Model file for the job. Use its own axes, mm. A direction names the side the tool comes from. Round coordinates to 2 decimals unless told otherwise and drop trailing zeros. Loops run counter-clockwise (first coordinate to the right, second up) from the corner with the lowest first, then second, coordinate; pieces in that order, holes last. Notation, with made-up numbers: M 61,-32.5 L 112,-32.5 A18 cw 112,-23.5 Z; hole C -19.5,52 d9. An arc over 180 degrees is marked long. Use a Markdown table: item, result. Add a question column.
Q1. Tool access for faces 1 (the face through (-1, 9, 75)), 2 (the face through (-1, 8, 77)): list every direction of +Z, -Z, +X, -X, +Y, -Y with a clear straight run to the whole face (end or side of a thin tool).
Q2. Cut at C-C (y = 5.5). Give the cut face in (x, z).
Q3. Cut at B-B (x = 31). Give the cut face in (y, z).
Q4. Probe line 1 (X direction, y = 15.5, z = 20.5); line 2 (Y direction, x = 62.5, z = 6). List the from-to ranges inside material, lowest first. Write a range as from..to.
Q5. Cut at A-A (z = -65.5). Give the cut face in (x, y), plus the area to 3 significant figures.
Q6. Mould opens along Z. For faces 3 (the face through (-1, 0, -1)), 4 (the face through (-1, 9, -75)), 5 (the face through (-1, 2, -1)), 6 (the face through (-1, 8, -77)) say: +Z half, -Z half, draft (parallel to the pull), parting line (faces both ways), or undercut.
from build123d import *

# Parameters (mm, degrees)
SKETCH1_W           = 150
SKETCH1_H           = 150
BOSS_EXTRUDE1_DEPTH = 2
SKETCH2_W           = 154
SKETCH2_H           = 154
BOSS_EXTRUDE2_DEPTH = 2
SKETCH3_W           = 154
SKETCH3_H           = 154
SKETCH3_W_2         = 150
SKETCH3_H_2         = 150
BOSS_EXTRUDE3_DEPTH = 15


with BuildPart() as part:
    # Sketch1 → Boss-Extrude1 (new body)
    with BuildSketch(Plane(origin=(0, 0, 0), x_dir=(1, 0, 0), z_dir=(0, 1, 0))):
        Rectangle(SKETCH1_W, SKETCH1_H)
    extrude(amount=BOSS_EXTRUDE1_DEPTH)

    # Sketch2 → Boss-Extrude2 (add)
    with BuildSketch(Plane(origin=(0, 2, 0), x_dir=(1, 0, 0), z_dir=(0, 1, 0))):
        Rectangle(SKETCH2_W, SKETCH2_H)
    extrude(amount=-BOSS_EXTRUDE2_DEPTH)

    # Sketch3 → Boss-Extrude3 (add)
    with BuildSketch(Plane(origin=(0, 2, 0), x_dir=(1, 0, 0), z_dir=(0, 1, 0))):
        Rectangle(SKETCH3_W, SKETCH3_H)
        Rectangle(SKETCH3_W_2, SKETCH3_H_2, mode=Mode.SUBTRACT)
    extrude(amount=BOSS_EXTRUDE3_DEPTH)


solid = part.part
Checked values:
| question | item | result |
|---|---|---|
| 1 | face 1 | +Y |
| 1 | face 2 | +Z, +X, -X, +Y, -Y |
| 2 | outline | M -77,-77 L 77,-77 L 77,77 L -77,77 Z; hole M -75,-75 L 75,-75 L 75,75 L -75,75 Z |
| 3 | outline | M 0,-77 L 17,-77 L 17,-75 L 2,-75 L 2,75 L 17,75 L 17,77 L 0,77 Z |
| 4 | line 1 | x = -77..-75, 75..77 |
| 4 | line 2 | y = 0..2 |
| 5 | outline | M -77,0 L 77,0 L 77,17 L 75,17 L 75,2 L -75,2 L -75,17 L -77,17 Z |
| 5 | area | 368 mm^2 |
| 6 | face 3 | draft |
| 6 | face 4 | undercut |
| 6 | face 5 | undercut |
| 6 | face 6 | -Z half |
